from build123d import *

# Parameters (mm, degrees)
SKETCH1_W           = 30
SKETCH1_H           = 30
SKETCH1_W_2         = 20
SKETCH1_H_2         = 20
BOSS_EXTRUDE2_DEPTH = 30
BOSS_EXTRUDE3_DEPTH = 30
SKETCH6_W           = 21
SKETCH6_H           = 55
CUT_EXTRUDE1_DEPTH  = 3
SKETCH7_R           = 1.5
CUT_EXTRUDE2_DEPTH  = 5
SKETCH8_W           = 21
SKETCH8_H           = 40.9
CUT_EXTRUDE3_DEPTH  = 3
SKETCH9_R           = 10.5
CUT_EXTRUDE4_DEPTH  = 81.056214629
BOSS_EXTRUDE4_START = -10
SKETCH10_R          = 10.5
SKETCH10_R_2        = 4
BOSS_EXTRUDE4_DEPTH = 10
FILLET1_R           = 10
SKETCH11_R          = 1.5
CUT_EXTRUDE5_DEPTH  = 81.175402093


with BuildPart() as part:
    # Sketch1 → Boss-Extrude2 (new body)
    with BuildSketch(Plane.XY):
        Rectangle(SKETCH1_W, SKETCH1_H)
        Rectangle(SKETCH1_W_2, SKETCH1_H_2, mode=Mode.SUBTRACT)
    extrude(amount=BOSS_EXTRUDE2_DEPTH)

    # Sketch5 → Boss-Extrude3 (add)
    with BuildSketch(Plane(origin=(0, 20.68, 0), x_dir=(1, 0, 0), z_dir=(0, 1, 0))):
        with BuildLine():
            Line((-15, -30.030941434), (-15, -0.030941434))
            ThreePointArc((-15, -0.030941434), (-35, 19.969058566), (-55, -0.030941434))
            Line((-55, -0.030941434), (-55, -30.030941434))
            ThreePointArc((-55, -30.030941434), (-35, -50.030941434), (-15, -30.030941434))
        make_face()
    extrude(amount=-BOSS_EXTRUDE3_DEPTH)

    # Sketch6 → Cut-Extrude1 (cut)
    with BuildSketch(Plane(origin=(0, 20.68, 0), x_dir=(1, 0, 0), z_dir=(0, 1, 0))):
        with Locations((-35, -15.030941434)):
            Rectangle(SKETCH6_W, SKETCH6_H)
    extrude(amount=-CUT_EXTRUDE1_DEPTH, mode=Mode.SUBTRACT)

    # Sketch7 → Cut-Extrude2 (cut)
    with BuildSketch(Plane(origin=(0, 17.68, 0), x_dir=(1, 0, 0), z_dir=(0, 1, 0))):
        with Locations(Location((-35, -39.030941434, 0), (0, 0, 270))):
            Circle(SKETCH7_R)
        with Locations(Location((-35, 8.969058566, 0), (0, 0, 270))):
            Circle(SKETCH7_R)
    extrude(amount=-CUT_EXTRUDE2_DEPTH, mode=Mode.SUBTRACT)

    # Sketch8 → Cut-Extrude3 (cut)
    with BuildSketch(Plane(origin=(0, 17.68, 0), x_dir=(1, 0, 0), z_dir=(0, 1, 0))):
        with Locations((-35, -15.030941434)):
            Rectangle(SKETCH8_W, SKETCH8_H)
    extrude(amount=-CUT_EXTRUDE3_DEPTH, mode=Mode.SUBTRACT)

    # Sketch9 → Cut-Extrude4 (cut, through all)
    with BuildSketch(Plane(origin=(0, 14.68, 0), x_dir=(1, 0, 0), z_dir=(0, 1, 0))):
        with Locations(Location((-35, -5.030941434, 0), (0, 0, 180))):
            Circle(SKETCH9_R)
    extrude(amount=-CUT_EXTRUDE4_DEPTH, mode=Mode.SUBTRACT)

    # Sketch10 → Boss-Extrude4 (add)
    with BuildSketch(Plane.XZ.offset(9.32).offset(BOSS_EXTRUDE4_START)):
        with Locations(Location((-35, 5.030941434, 0), (0, 0, 180))):
            Circle(SKETCH10_R)
        with Locations(Location((-35, 5.030941434, 0), (0, 0, 270))):
            Circle(SKETCH10_R_2, mode=Mode.SUBTRACT)
    extrude(amount=BOSS_EXTRUDE4_DEPTH)

    # Fillet1
    # the kernel refuses this fillet: 10 mm, written as the material it adds along each edge
    with BuildSketch(Plane(origin=(-15, 15, -22.515898699), x_dir=(1, 0, 0), z_dir=(0, 0, 1))) as fillet1_piece_1_section:
        with BuildLine():
            CenterArc((9.018736053, 10), FILLET1_R, 205.594552278, 64.405447722)
            Line((0, 5.68), (0, 0))
            Line((0, 0), (9.018736053, 0))
        make_face()
    fillet1_piece_1 = extrude(amount=52.515898699, mode=Mode.PRIVATE)
    fillet1_piece_1 = split(fillet1_piece_1, bisect_by=Plane(origin=(-11.321087315, 16.521398323, 0), z_dir=(0, 0, 1)), keep=Keep.TOP, mode=Mode.PRIVATE)
    add(fillet1_piece_1)

    # Sketch11 → Cut-Extrude5 (cut, through all)
    with BuildSketch(Plane(origin=(0, 15, 0), x_dir=(1, 0, 0), z_dir=(0, 1, 0))):
        with Locations(Location((0, -15, 0), (0, 0, 270))):
            Circle(SKETCH11_R)
    extrude(amount=-CUT_EXTRUDE5_DEPTH, mode=Mode.SUBTRACT)


solid = part.part
Could you check a few things on this model? Use its own coordinates, in mm. A direction names the side the tool comes from. Round coordinates to 2 decimals unless told otherwise and drop trailing zeros. Order: outer loops, then holes, each group sorted by start corner. A loop starts at its lowest first (then second) coordinate and runs counter-clockwise, first axis right, second up.
Q1. I'm going to push flat-ended pins straight in: P1, Ø2.5, axis at x = -35, z = -8.5, coming from the +Y side; P2, Ø6.5, axis at x = 3, z = 19, coming from the +Y side; P3, Ø1, axis at x = -42.5, z = 25, coming from the +Y side. Where does each tip first touch, or does it pass through?
Geometry says:
P1: stops at y = 17.68
P2: stops at y = 15
P3: stops at y = 14.68
Q2. Imagine slicing it at B-B, the plane x = -35. List the corners of the cut face in (y, z) for me.
Geometry says:
outline: (-9.32, -19.97) - (20.68, -19.97) - (20.68, -12.47) - (17.68, -12.47) - (17.68, -10.47) - (12.68, -10.47) - (12.68, -7.47) - (17.68, -7.47) - (17.68, -5.42) - (14.68, -5.42) - (14.68, -5.47) - (0.68, -5.47) - (0.68, 1.03) - (-9.32, 1.03) - close; (-9.32, 9.03) - (0.68, 9.03) - (0.68, 15.53) - (14.68, 15.53) - (14.68, 35.48) - (17.68, 35.48) - (17.68, 37.53) - (12.68, 37.53) - (12.68, 40.53) - (17.68, 40.53) - (17.68, 42.53) - (20.68, 42.53) - (20.68, 50.03) - (-9.32, 50.03) - close
Q3. Please list where these lines run through material, in increasing order: probe 1 along Y at (x, z) = (5, 12); probe 2 along X at (y, z) = (4.5, 21.5); probe 3 along Y at (x, z) = (-32, 41).
Geometry says:
probe 1: y = -15 to -10, 10 to 15
probe 2: x = -55 to -10, 10 to 15
probe 3: y = -9.32 to 17.68
Q4. Imagine slicing it at A-A, the plane y = -1. State how many separate pieces and enclosed holes the cut face has, then the cut area to 3 significant figures.
Geometry says:
separate pieces: 2
enclosed holes: 1
area: 2,710 mm2
Q5. Imagine slicing it at C-C, the plane z = 20. List the corners of the cut face in (x, y) for me.
Geometry says:
outline: (-55, -9.32) - (-15, -9.32) - (-15, -15) - (15, -15) - (15, 15) - (-5.98, 15) arc R10 cw to (-15, 20.68) - (-24.5, 20.68) - (-24.5, 14.68) - (-45.5, 14.68) - (-45.5, 20.68) - (-55, 20.68) - close; hole (-10, -10) - (10, -10) - (10, 10) - (-10, 10) - close
Q6. Which directions (+Z, -Z, +X, -X, +Y, -Y) give clear straight access to the entire face, cutting with the end or side of a thin tool? Please do faces 1 (the face through (-31.034, -4.25, 5.552)), 2 (the face through (-27, 14.68, -3)), 3 (the face through (10, 0, 15)), 4 (the face through (4, 15, 15)).
Geometry says:
face 1: +Y, -Y
face 2: +Y
face 3: +Z, -Z
face 4: +Z, -Z, +X, +Y
Q7. Imagine slicing it at D-D, the plane x = 0. List the corners of the cut face in (y, z) for me.
Geometry says:
outline: (-15, 0) - (-10, 0) - (-10, 13.5) - (-15, 13.5) - close; (-15, 16.5) - (-10, 16.5) - (-10, 30) - (-15, 30) - close; (10, 0) - (15, 0) - (15, 13.5) - (10, 13.5) - close; (10, 16.5) - (15, 16.5) - (15, 30) - (10, 30) - close
Q8. Thinking about a two-plate mould opening in Y: for faces 5 (the face through (-22, 20.68, 15)), 6 (the face through (-36.331, 15.215, -8.277)), 7 (the face through (2, 10, 15)), which applies, released by +Y, released by -Y, zero draft, split by the parting line, or undercut?
Geometry says:
face 5: released by +Y
face 6: zero draft
face 7: undercut
